Part model, mm, in its own coordinate system. A direction names the side the tool comes from. Coordinates: 2 decimals unless noted, no trailing zeros. Loops run counter-clockwise (first coordinate to the right, second up) from the corner with the lowest first, then second, coordinate; pieces in that order, holes last. Notation, with made-up numbers: M -14.75,-13 L 24.25,-13 A22 ccw 24.25,13 Z; hole C 23.25,29.5 d5. An arc over 180 degrees is marked long. Use a Markdown table: item, result. Add a question column.
1) Band-saw the part on C-C (z = -35.5). List the corners of the cut face in (x, y), plus the area to 3 significant figures.
2) Tool access for faces 4 (the flat face through (40, 26, 0)), 5 (the cylindrical face through (46.37, 10.3, -5.07)): list every direction of +Z, -Z, +X, -X, +Y, -Y with a clear straight run to the whole face (end or side of a thin tool).
3) Wall check: probe 1 along Y at (x, z) = (0, -35); probe 2 along Y at (x, z) = (0, -6.75); probe 3 along X at (y, z) = (-26.5, -83). Give the ranges that are in metal, low to high. Write a range as from..to.
4) Pin check, flat tips, straight feed: pin 1 Ø1 at (y, z) = (-26.5, -43) entering from -X; pin 2 Ø1.5 at (y, z) = (-2.5, -112.5) entering from -X; pin 3 Ø8 at (x, z) = (-1, -73) entering from +Y. Stop position of each tip, or through.
5) Band-saw the part on A-A (y = 0). List the corners of the cut face in (x, z).
6) Pull direction Y, two halves, no side cores. Call faces 1 (the flat face through (0, -50, -134)), 2 (the cylindrical face through (-51.73, -21.45, -138.06)), 3 (the cylindrical face through (-45.61, 5.99, -76.92)): released by +Y, released by -Y, zero draft, split by the parting line, or undercut.
Autodesk Inventor part; units mm, degrees
ref_plane "YZ Plane" through (0, 0, 0) normal (1, 0, 0) x (0, 1, 0)
ref_plane "XZ Plane" through (0, 0, 0) normal (0, 1, 0) x (-1, 0, 0)
ref_plane "XY Plane" through (0, 0, 0) normal (0, 0, 1) x (1, 0, 0)
sketch "Skizze1" plane through (0, 0, 0) normal (0, 1, 0) x (-1, 0, 0)
  line L0 (0, 0) -> (0, -142)
  line L1 (0, 0) -> (49, 0)
  line L2 (49, 0) -> (49, -134)
  line L3 (49, -134) -> (56, -134)
  line L4 (56, -134) -> (56, -142)
  line L5 (56, -142) -> (0, -142)
  dimension "d0" = 112
  dimension "d1" = 8
  dimension "d2" = 134
  dimension "d3" = 98
revolve "Umdrehung1" add sketch "Skizze1" angle 360 about axis through (0, 0, 0) along (0, 0, -1)
sketch "Skizze2" plane through (0, 0, 0) normal (0, 0, 1) x (1, 0, 0)
  circle A0 centre (0, 0) radius 49
hole "Bohrung1" at (0, 0, 0) direction (0, 0, -1) diameter 92 end through all counterbore diameter 95 counterbore depth 10
properties part number "13" material "Phenolharz"
Entries:
| question | item | result |
|---|---|---|
| 1 | outline | C 0,0 d98; hole C 0,0 d92 |
| 1 | area | 895 mm2 |
| 2 | face 4 | +Z, +X, -X, +Y, -Y |
| 2 | face 5 | +Z |
| 3 | probe 1 | -49..-46, 46..49 |
| 3 | probe 2 | -49..-47.5, 47.5..49 |
| 3 | probe 3 | -41.22..-37.6, 37.6..41.22 |
| 4 | pin 1 | x = -41.53 |
| 4 | pin 2 | x = -48.97 |
| 4 | pin 3 | y = 49 |
| 5 | outline | M -56,-142 L -46,-142 L -46,-10 L -47.5,-10 L -47.5,0 L -49,0 L -49,-134 L -56,-134 Z; M 46,-142 L 56,-142 L 56,-134 L 49,-134 L 49,0 L 47.5,0 L 47.5,-10 L 46,-10 Z |
| 6 | face 1 | zero draft |
| 6 | face 2 | split by the parting line |
| 6 | face 3 | undercut |
